```python
from build123d import *

# Parameters (mm, degrees)
SKETCH_1_R          = 2.0955
EXTRUDE_1_DEPTH     = 1.5
SKETCH_2_R          = 2.1
CUT_EXTRUDE_1_DEPTH = 1.5
FILLET_1_R          = 6
CUT_EXTRUDE_START   = -1.5
SKETCH_3_W          = 25.639754975
SKETCH_3_H          = 15.572778706
SKETCH_3_R          = 2.0955
CUT_EXTRUDE_3_DEPTH = 1.5
FILLET_2_R          = 4


with BuildPart() as part:
    # 草图1 → 凸台-拉伸1 (new body)
    with BuildSketch(Plane(origin=(0, 0, 0), x_dir=(1, 0, 0), z_dir=(0, 1, 0))):
        with BuildLine():
            Line((-105.503818672, 6.037520304), (-105.503818672, -35.395112744))
            Line((-105.503818672, -35.395112744), (44.496181328, -35.395112744))
            Line((44.496181328, -35.395112744), (44.496181328, 6.037520304))
            Line((44.496181328, 6.037520304), (-14.469645921, 60.536135507))
            ThreePointArc((-14.469645921, 60.536135507), (-20.755816559, 64.47318161), (-28.044474141, 65.848588442))
            Line((-28.044474141, 65.848588442), (-33.461010911, 65.848588442))
            ThreePointArc((-33.461010911, 65.848588442), (-40.789042153, 64.457724857), (-47.097844214, 60.478584254))
            Line((-47.097844214, 60.478584254), (-105.503818672, 6.037520304))
        make_face()
        with Locations(Location((-94.003818672, -29.045112744, 0), (0, 0, 270))):
            Circle(SKETCH_1_R, mode=Mode.SUBTRACT)
        with Locations(Location((32.996181328, -29.045112744, 0), (0, 0, 270))):
            Circle(SKETCH_1_R, mode=Mode.SUBTRACT)
        with Locations(Location((-68.603818672, -29.045112744, 0), (0, 0, 270))):
            Circle(SKETCH_1_R, mode=Mode.SUBTRACT)
        with Locations(Location((-43.203818672, -29.045112744, 0), (0, 0, 270))):
            Circle(SKETCH_1_R, mode=Mode.SUBTRACT)
        with Locations(Location((-17.803818672, -29.045112744, 0), (0, 0, 270))):
            Circle(SKETCH_1_R, mode=Mode.SUBTRACT)
        with Locations(Location((7.596181328, -29.045112744, 0), (0, 0, 270))):
            Circle(SKETCH_1_R, mode=Mode.SUBTRACT)
    extrude(amount=EXTRUDE_1_DEPTH)

    # 草图2 → 切除-拉伸1 (cut)
    with BuildSketch(Plane(origin=(0, 1.5, 0), x_dir=(1, 0, 0), z_dir=(0, 1, 0))):
        with Locations(Location((-81.303818672, -29.045112744, 0), (0, 0, 270))):
            Circle(SKETCH_2_R)
        with Locations(Location((20.296181328, -29.045112744, 0), (0, 0, 270))):
            Circle(SKETCH_2_R)
        with Locations(Location((-94.655027928, 5.896929075, 0), (0, 0, 270))):
            Circle(SKETCH_2_R)
        with Locations(Location((-76.078643907, 23.219687421, 0), (0, 0, 270))):
            Circle(SKETCH_2_R)
        with Locations(Location((-57.502259886, 40.542445766, 0), (0, 0, 270))):
            Circle(SKETCH_2_R)
        with Locations(Location((-38.925875865, 57.865204112, 0), (0, 0, 270))):
            Circle(SKETCH_2_R)
        with Locations(Location((33.647390585, 5.896929075, 0), (0, 0, 90))):
            Circle(SKETCH_2_R)
        with Locations(Location((15.071006563, 23.219687421, 0), (0, 0, 90))):
            Circle(SKETCH_2_R)
        with Locations(Location((-3.505377458, 40.542445766, 0), (0, 0, 90))):
            Circle(SKETCH_2_R)
        with Locations(Location((-22.081761479, 57.865204112, 0), (0, 0, 90))):
            Circle(SKETCH_2_R)
    extrude(amount=-CUT_EXTRUDE_1_DEPTH, mode=Mode.SUBTRACT)

    # 圆角1
    fillet_1_edges = [part.edges().sort_by_distance(p)[0] for p in [
        (44.496181328, 0.75, -6.037520304),
        (44.496181328, 0.75, 35.395112744),
        (-105.503818672, 0.75, 35.395112744),
        (-105.503818672, 0.75, -6.037520304),
    ]]
    fillet(fillet_1_edges, radius=FILLET_1_R)

    # 草图3 → 切除-拉伸3 (cut)
    # profile 1 of 2: a face of its own
    with BuildSketch(Plane(origin=(0, 1.5, 0), x_dir=(1, 0, 0), z_dir=(0, 1, 0)).offset(CUT_EXTRUDE_START)):
        with Locations((-64.205559978, -27.608723391)):
            Rectangle(SKETCH_3_W, SKETCH_3_H)
        with Locations((-68.603818672, -29.045112744)):
            Circle(SKETCH_3_R, mode=Mode.SUBTRACT)
    # profile 2 of 2: a face of its own
    with BuildSketch(Plane(origin=(0, 1.5, 0), x_dir=(1, 0, 0), z_dir=(0, 1, 0)).offset(CUT_EXTRUDE_START)):
        with Locations((3.197922635, -27.608723391)):
            Rectangle(SKETCH_3_W, SKETCH_3_H)
        with Locations((7.596181328, -29.045112744)):
            Circle(SKETCH_3_R, mode=Mode.SUBTRACT)
    extrude(amount=CUT_EXTRUDE_3_DEPTH, mode=Mode.SUBTRACT)

    # 圆角2
    fillet_2_edges = [part.edges().sort_by_distance(p)[0] for p in [
        (-51.38568249, 0.75, 35.395112744),
        (-77.025437465, 0.75, 35.395112744),
        (-77.025437465, 0.75, 19.822334038),
        (-51.38568249, 0.75, 19.822334038),
        (16.017800122, 0.75, 35.395112744),
        (-9.621954853, 0.75, 35.395112744),
        (-9.621954853, 0.75, 19.822334038),
        (16.017800122, 0.75, 19.822334038),
    ]]
    fillet(fillet_2_edges, radius=FILLET_2_R)


solid = part.part
```
Work out the finished part from the listing and answer in its coordinate system (mm). A direction names the side the tool comes from. Coordinates: 2 decimals unless noted, no trailing zeros. Loops run counter-clockwise (first coordinate to the right, second up) from the corner with the lowest first, then second, coordinate; pieces in that order, holes last. Notation, with made-up numbers: M -24,40.5 L -1,40.5 A12 ccw -1,46.5 Z; hole C 83,-35.75 d5. An arc over 180 degrees is marked long. Use CSV: the item, a comma, the result in double quotes. Start each with the question number.
(1) Find section B-B, the plane y = 0.8. State how many separate pieces and enclosed holes the cut face has, then the cut area to 3 significant figures.
(2) Find section A-A, the plane z = -40. Give the vertices of the cut face in (x, y).
(3) Consider line 1 (X direction, y = 0.3, z = -21.5); line 2 (X direction, y = 0.7, z = 23); line 3 (Z direction, x = -39.5, y = 1.3). Determine where each line is inside the solid, lowest interval first.
(4) For a pull along Z with two mould halves and no side action, classify faces 3 (the face through (-23.852, 0.76, -58.994)), 4 (the face through (-74.951, 0.74, -34.516)), 5 (the face through (-5.588, 0.76, -40.269)), 6 (the face through (17.221, 0.76, 34.254)) as +Z half, -Z half, draft (parallel to the pull), parting line (faces both ways), or undercut.
(5) Find section D-D, the plane z = -10. Give the vertices of the cut face in (x, y).
(6) For faces 1 (the face through (-37.155, 0.76, -56.736)), 2 (the face through (-10.76, 0.76, 34.19)), determine the directions among +Z, -Z, +X, -X, +Y, -Y from which every point of the face is accessible in a straight line to the end or side of a thin tool.
(7) Find section C-C, the plane z = -54. Give the vertices of the cut face in (x, y).
Recorded:
1,separate pieces,"1"
1,enclosed holes,"14"
1,area,"10,300 mm^2"
2,outline,"M -69.07,0 L -59.53,0 L -59.53,1.5 L -69.07,1.5 Z; M -55.47,0 L -5.53,0 L -5.53,1.5 L -55.47,1.5 Z; M -1.48,0 L 7.75,0 L 7.75,1.5 L -1.48,1.5 Z"
3,line 1,"x = -88.92 to -77.28, -74.87 to 13.87, 16.28 to 27.77"
3,line 2,"x = -105.5 to -76.94, -51.47 to -9.54, 15.93 to 44.5"
3,line 3,"z = -64.92 to -59.89, -55.85 to 35.4"
4,face 3,"undercut"
4,face 4,"-Z half"
4,face 5,"undercut"
4,face 6,"+Z half"
5,outline,"M -101.25,0 L 40.21,0 L 40.21,1.5 L -101.25,1.5 Z"
6,face 1,"+Y, -Y"
6,face 2,"+Z, +Y, -Y"
7,outline,"M -54.05,0 L -7.4,0 L -7.4,1.5 L -54.05,1.5 Z"
